Here's how the part is built. I have some questions about the finished solid (model axes, mm). Face numbers are marked on the shaded views. A direction names the side the tool comes from. Give positions to 0.01 mm unless a question says otherwise; leave off trailing zeros. Write each loop counter-clockwise with the first axis right and the second up, starting at its lowest first coordinate (ties: lowest second). Pieces come first, ordered by that corner, then holes. Notation, with made-up numbers: (2, 57.25) - (31, 57.25) arc R31 cw to (31, 89.25) - close; hole circle Ø6 at (-38.75, 17.25). An arc over 180 degrees is marked (long way). Use one line per item in the form item = value. Start each with the question number.
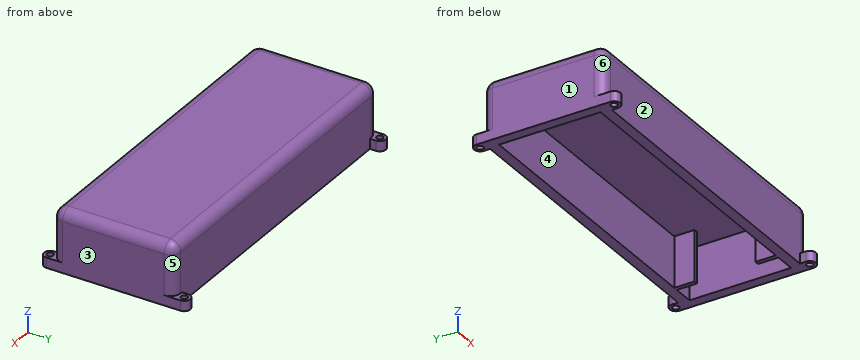
from build123d import *

# Parameters (mm, degrees)
SKETCH1_W                 = 5
SKETCH1_H                 = 50
SKETCH1_H_2               = 60
SKETCH1_W_2               = 2
SKETCH1_H_3               = 10
BOSS_EXTRUDE1_DEPTH       = 25
SKETCH2_W                 = 160
SKETCH2_H                 = 60
BOSS_EXTRUDE2_DEPTH       = 5
SKETCH5_R                 = 3
SKETCH5_R_2               = 1.6
BOSS_EXTRUDE3_DEPTH       = 5
MIRROR2_COPY_1_SKETCH_R   = 3
MIRROR2_COPY_1_SKETCH_R_2 = 1.6
MIRROR2_COPY_1_DEPTH      = 5
FILLET1_R                 = 5


with BuildPart() as part:
    # Sketch1 → Boss-Extrude1 (new body)
    with BuildSketch(Plane.XY):
        with Locations((77.5, 0)):
            Rectangle(SKETCH1_W, SKETCH1_H)
        Polygon((-75, -25), (-75, -30), (80, -30), (80, -25), (75, -25), (65, -25), (63, -25), align=None)
        with Locations((-77.5, 0)):
            Rectangle(SKETCH1_W, SKETCH1_H_2)
        Polygon((80, 30), (-75, 30), (-75, 25), (63, 25), (65, 25), (75, 25), (80, 25), align=None)
        with Locations((64, -20)):
            Rectangle(SKETCH1_W_2, SKETCH1_H_3)
        with Locations((64, 20)):
            Rectangle(SKETCH1_W_2, SKETCH1_H_3)
    extrude(amount=BOSS_EXTRUDE1_DEPTH)

    # Sketch2 → Boss-Extrude2 (add)
    with BuildSketch(Plane.XY.offset(25)):
        Rectangle(SKETCH2_W, SKETCH2_H)
    extrude(amount=BOSS_EXTRUDE2_DEPTH)

    # Sketch5 → Boss-Extrude3 (add)
    with BuildSketch(Plane(origin=(0, 0, 0), x_dir=(-1, 0, 0), z_dir=(0, 0, -1))):
        with Locations((77, -33)):
            Circle(SKETCH5_R)
        with Locations((77, -33)):
            Circle(SKETCH5_R_2, mode=Mode.SUBTRACT)
        with BuildLine():
            ThreePointArc((77, -30), (79.121320344, -30.878679656), (80, -33))
            Line((80, -33), (80, -30))
            Line((80, -30), (77, -30))
        make_face()
        with BuildLine():
            Line((74, -30), (74, -33))
            ThreePointArc((74, -33), (74.878679656, -30.878679656), (77, -30))
            Line((77, -30), (74, -30))
        make_face()
    boss_extrude3 = extrude(amount=-BOSS_EXTRUDE3_DEPTH)

    # Mirror1: Boss-Extrude3 across plane
    add(boss_extrude3.mirror(Plane(origin=(0, 0, 0), x_dir=(0, 0, 1), z_dir=(1, 0, 0))))

    # Mirror2: Boss-Extrude3 across plane
    add(boss_extrude3.mirror(Plane.ZX))

    # Mirror2 copy 1 sketch → Mirror2 copy 1 (add)
    with BuildSketch(Plane(origin=(0, 0, 0), x_dir=(1, 0, 0), z_dir=(0, 0, -1))):
        with Locations((77, -33)):
            Circle(MIRROR2_COPY_1_SKETCH_R)
        with Locations((77, -33)):
            Circle(MIRROR2_COPY_1_SKETCH_R_2, mode=Mode.SUBTRACT)
        with BuildLine():
            ThreePointArc((77, -30), (79.121320344, -30.878679656), (80, -33))
            Line((80, -33), (80, -30))
            Line((80, -30), (77, -30))
        make_face()
        with BuildLine():
            Line((74, -30), (74, -33))
            ThreePointArc((74, -33), (74.878679656, -30.878679656), (77, -30))
            Line((77, -30), (74, -30))
        make_face()
    extrude(amount=-MIRROR2_COPY_1_DEPTH)

    # Fillet1
    fillet1_edges = [part.edges().sort_by_distance(p)[0] for p in [
        (-80, 30, 17.5),
        (80, 30, 17.5),
        (80, -30, 17.5),
        (-80, -30, 17.5),
        (0, 30, 30),
        (-80, 0, 30),
        (0, -30, 30),
        (80, 0, 30),
    ]]
    fillet(fillet1_edges, radius=FILLET1_R)


solid = part.part
1. For the marked faces 4, 5 and 6, which set-ups out of +Z, -Z, +X, -X, +Y, -Y let a thin tool reach every point of the face, with its end or its side?
2. For P1, Ø3, axis at x = -42, z = 18, coming from the -Y side; P2, Ø1, axis at x = 4, y = -1, coming from the -Z side; P3, Ø5, axis at x = -62.5, z = 7, coming from the +Y side, each with a flat end and sliding along its axis, tell me the tip position at first contact or that it passes through.
3. We'd pull the mould along X, two halves only. Please class the marked faces 1, 2 and 3: pulls with the +X half, pulls with the -X half, needs draft (parallel to the pull), parting line crosses it, or undercut.
4. I want a section at A-A, the plane x = -77. List the corners of the cut face in (y, z) for me, then the cut area to 3 significant figures.
5. Please list where these lines run through material, in increasing order: line 1 (X direction, y = -23, z = 18); line 2 (Y direction, x = 77, z = 1.55); line 3 (X direction, y = 33, z = 3.6).
6. I want a section at C-C, the plane y = 20.5. List the corners of the cut face in (x, z) for me, then the cut area to 3 significant figures.
7. I want a section at D-D, the plane x = -27. List the corners of the cut face in (y, z) for me.
8. I want a section at B-B, the plane z = 8.75. List the corners of the cut face in (x, y) for me, then the cut area to 3 significant figures.
Result sheet:
q1.face_4 = -Z
q1.face_5 = +Z, +X, +Y
q1.face_6 = +Z, -X, -Y
q2.P1 = -30
q2.P2 = 25
q2.P3 = 30
q3.face_1 = pulls with the -X half
q3.face_2 = undercut
q3.face_3 = pulls with the +X half
q4.outline = (-36, 0) - (-34.6, 0) - (-34.6, 5) - (-36, 5) - close; (-31.4, 0) - (31.4, 0) - (31.4, 5) - (29.58, 5) - (29.58, 25) arc R4.58 ccw to (25, 29.58) - (-25, 29.58) arc R4.58 ccw to (-29.58, 25) - (-29.58, 5) - (-31.4, 5) - close; (34.6, 0) - (36, 0) - (36, 5) - (34.6, 5) - close
q4.area = 1,770 mm2
q5.line_1 = -80 to -75, 63 to 65, 75 to 80
q5.line_2 = -36 to -34.6, -31.4 to 31.4, 34.6 to 36
q5.line_3 = -80 to -78.6, -75.4 to -74, 74 to 75.4, 78.6 to 80
q6.outline = (-80, 0) - (-75, 0) - (-75, 25) - (63, 25) - (63, 0) - (65, 0) - (65, 25) - (75, 25) - (75, 0) - (80, 0) - (80, 25) arc R5 ccw to (75, 30) - (-75, 30) arc R5 ccw to (-80, 25) - close
q6.area = 1,090 mm2
q7.outline = (-30, 0) - (-25, 0) - (-25, 25) - (25, 25) - (25, 0) - (30, 0) - (30, 25) arc R5 ccw to (25, 30) - (-25, 30) arc R5 ccw to (-30, 25) - close
q8.outline = (-80, -25) arc R5 ccw to (-75, -30) - (75, -30) arc R5 ccw to (80, -25) - (80, 25) arc R5 ccw to (75, 30) - (-75, 30) arc R5 ccw to (-80, 25) - close; hole (-75, -25) - (63, -25) - (63, -15) - (65, -15) - (65, -25) - (75, -25) - (75, 25) - (65, 25) - (65, 15) - (63, 15) - (63, 25) - (-75, 25) - close
q8.area = 2,120 mm2
